from build123d import *

# Parameters (mm, degrees)
SKETCH1_W           = 215
SKETCH1_H           = 160
BOSS_EXTRUDE1_DEPTH = 3
SKETCH2_R           = 1.35
SKETCH2_R_2         = 1
SKETCH2_R_3         = 2.125
CUT_EXTRUDE1_DEPTH  = 4
FILLET1_R           = 10


with BuildPart() as part:
    # Sketch1 → Boss-Extrude1 (new body)
    with BuildSketch(Plane(origin=(0, 210, 0), x_dir=(1, 0, 0), z_dir=(0, 1, 0))):
        Rectangle(SKETCH1_W, SKETCH1_H)
    extrude(amount=BOSS_EXTRUDE1_DEPTH)

    # Sketch2 → Cut-Extrude1 (cut, through all)
    with BuildSketch(Plane(origin=(0, 213, 0), x_dir=(1, 0, 0), z_dir=(0, 1, 0))):
        with Locations((-78, -13.5)):
            Circle(SKETCH2_R)
        with Locations((-29, -13.5)):
            Circle(SKETCH2_R)
        with Locations((-29, -71.5)):
            Circle(SKETCH2_R)
        with Locations((-78, -71.5)):
            Circle(SKETCH2_R)
        with Locations((86.5, 14.5)):
            Circle(SKETCH2_R)
        with Locations((86.5, -71.5)):
            Circle(SKETCH2_R)
        with Locations((28.5, -71.5)):
            Circle(SKETCH2_R)
        with Locations((28.5, 14.5)):
            Circle(SKETCH2_R)
        with Locations((-78, 70)):
            Circle(SKETCH2_R)
        with Locations((-78, 25.55)):
            Circle(SKETCH2_R)
        with Locations((17.25, 25.55)):
            Circle(SKETCH2_R)
        with Locations((17.25, 70)):
            Circle(SKETCH2_R)
        with Locations((52.25, 54.5)):
            Circle(SKETCH2_R_2)
        with Locations((65.95, 54.5)):
            Circle(SKETCH2_R_2)
        with Locations((97.5, -70)):
            Circle(SKETCH2_R_3)
        with Locations((97.5, 70)):
            Circle(SKETCH2_R_3)
        with Locations((-97.5, 70)):
            Circle(SKETCH2_R_3)
        with Locations((-97.5, -70)):
            Circle(SKETCH2_R_3)
    extrude(amount=-CUT_EXTRUDE1_DEPTH, mode=Mode.SUBTRACT)

    # Fillet1
    fillet1_edges = [part.edges().sort_by_distance(p)[0] for p in [
        (-107.5, 211.5, -80),
        (107.5, 211.5, -80),
        (107.5, 211.5, 80),
        (-107.5, 211.5, 80),
    ]]
    fillet(fillet1_edges, radius=FILLET1_R)


solid = part.part
Design review of the part built by this model. Coordinates are the model's own, in mm. Coordinates: 2 decimals unless noted, no trailing zeros. Use one line per item in the form item = value.
Q1. Insertion check: pin 1 Ø2 at (x, z) = (86.5, 71.5) entering from +Y. The pin has a flat end and moves straight along its axis. Give the tip position at first contact, or say it passes through.
Taken from the geometry:
pin_1 = through
Q2. For probe 1 along Z at (x, y) = (17.25, 211.3); probe 2 along Z at (x, y) = (28.5, 210.8); probe 3 along Z at (x, y) = (52.25, 211), list the stretches that pass through material, from the lowest coordinate up.
Taken from the geometry:
probe_1 = -80 to -71.35, -68.65 to -26.9, -24.2 to 80
probe_2 = -80 to -15.85, -13.15 to 70.15, 72.85 to 80
probe_3 = -80 to -55.5, -53.5 to 80
Q3. The part is to be moulded in two halves that separate along X. For faces 1 (the cylindrical face through (-99.1, 211.5, -71.4)), 2 (the cylindrical face through (-104.65, 211.52, -76.99)), 3 (the cylindrical face through (104.49, 211.52, 77.15)), 4 (the cylindrical face through (95.9, 211.5, -71.4)), say which applies: +X half, -X half, draft (parallel to the pull), parting line (faces both ways), or undercut.
Taken from the geometry:
face_1 = undercut
face_2 = -X half
face_3 = +X half
face_4 = undercut
